Answer from the drawing. Dimensions are ordinates in mm from the lowest x, y and z of the part. A direction names the side the tool comes from. Round coordinates to 2 decimals unless told otherwise and drop trailing zeros. Loops run counter-clockwise (first coordinate to the right, second up) from the corner with the lowest first, then second, coordinate; pieces in that order, holes last. Notation, with made-up numbers: (-13, -30.75) - (38, -30.75) arc R29 cw to (38, 3.25) - close; hole circle Ø9 at (9.25, 54). An arc over 180 degrees is marked (long way). Return JSON: item names as keys, results as strings.
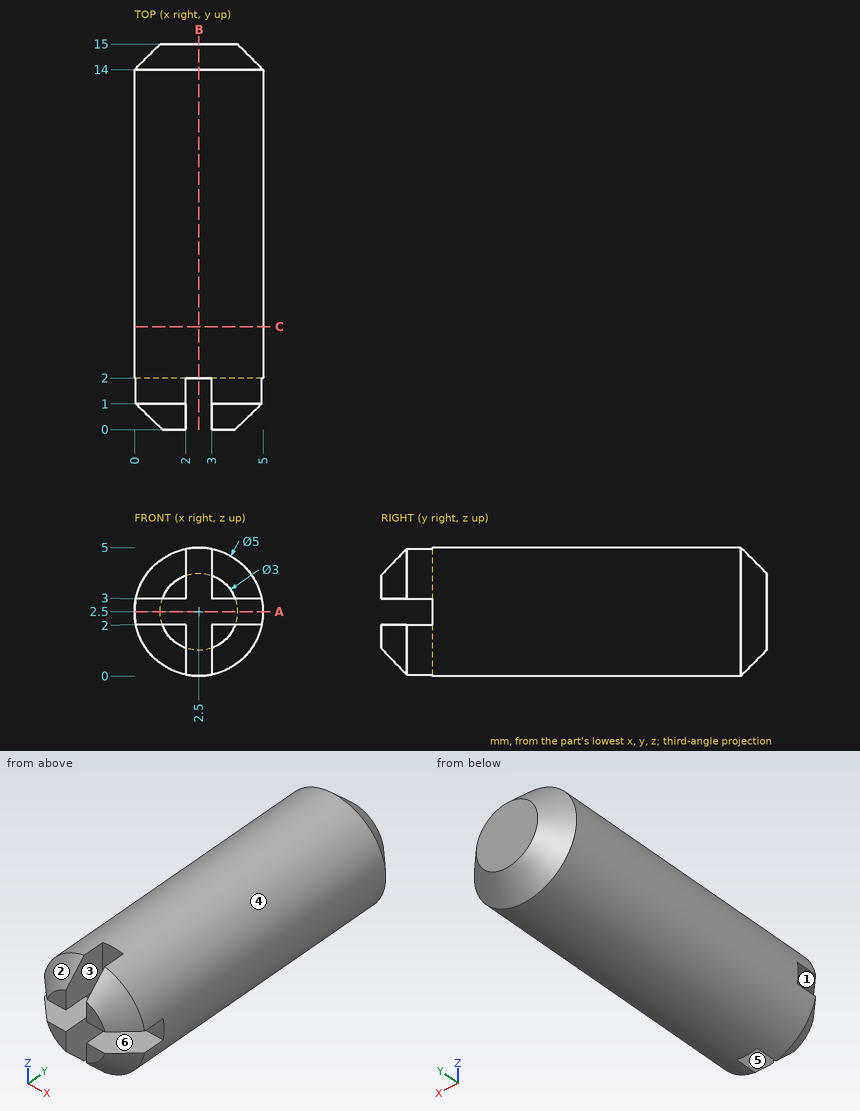
1) Section C-C (y = 4) is taken. Give the vertices of the cut face in (x, z).
Verdict:
{"outline": "circle Ø5 at (2.5, 2.5)"}
2) Section A-A (z = 2.5) is taken. Give the vertices of the cut face in (x, y), and give its area (3 significant figures).
Verdict:
{"outline": "(0, 2) - (5, 2) - (5, 14) - (4, 15) - (1, 15) - (0, 14) - close", "area": "64.0 mm2"}
3) Find the intervals of material crossed by L1, parallel to X at y = 11.5, z = 3; L2, parallel to X at y = 1.25, z = 4.2; L3, parallel to Y at x = 2.6, z = 1.15, in increasing order.
Verdict:
{"L1": "x = 0.05 to 4.95", "L2": "x = 0.67 to 2, 3 to 4.33", "L3": "y = 2 to 15"}
4) Flat-ended cylindrical pins translate along their axes: pin 1 (1.5 mm diameter, centred on x = 2.5, z = 2.5, fed in from -Y); pin 2 (1 mm diameter, centred on y = 1, z = 4.5, fed in from +X); pin 3 (1 mm diameter, centred on y = 1, z = 1, fed in from -X); pin 4 (1 mm diameter, centred on x = 4, y = 1, fed in from -Z). Find the tip coordinate at first contact, or state that the pin passes through.
Verdict:
{"pin 1": "stops at y = 0", "pin 2": "stops at x = 4.5", "pin 3": "stops at x = 0.21", "pin 4": "stops at z = 0.21"}
5) Determine the mould class of the marked faces 4, 5 and 6 for opening direction X: pulls with the +X half, pulls with the -X half, needs draft (parallel to the pull), parting line crosses it, or undercut.
Verdict:
{"face 4": "parting line crosses it", "face 5": "undercut", "face 6": "needs draft"}
6) Section B-B (x = 2.5) is taken. Give the vertices of the cut face in (y, z).
Verdict:
{"outline": "(2, 0) - (14, 0) - (15, 1) - (15, 4) - (14, 5) - (2, 5) - close"}
7) A tool of negligible diameter and unlimited length cuts with its end or side. For the marked faces 1, 2 and 3, from which of +Z, -Z, +X, -X, +Y, -Y can it reach the whole face along a straight path? Write none if from no direction.
Verdict:
{"face 1": "+X, -X, -Y", "face 2": "+Z, -X, -Y", "face 3": "+Z, -Z, -Y"}
